Model file for the job. Use its own axes, mm. A direction names the side the tool comes from. Give positions to 0.01 mm unless a question says otherwise; leave off trailing zeros. Loops run counter-clockwise (first coordinate to the right, second up) from the corner with the lowest first, then second, coordinate; pieces in that order, holes last. Notation, with made-up numbers: (78, 2.5) - (128, 2.5) arc R12 ccw to (128, 21.5) - close; hole circle Ø4 at (52.25, -16.5). An arc over 180 degrees is marked (long way). Answer as CSV lines item,"result". Start each with the question number.
Item 1: Saw through at A-A on z = 9. Give the cut face in (x, y), plus the area to 3 significant figures.
Item 2: Drill centre lines: L1, parallel to X at y = 1.05, z = 15.99; L2, parallel to X at y = 6.5, z = -15.5; L3, parallel to Z at x = -8.65, y = 6.2. Where is each one in solid material? Low to high. Write a range as from..to.
Item 3: Saw through at D-D on y = 5.5. State how many separate pieces and enclosed holes the cut face has, plus the area to 3 significant figures.
Item 4: Saw through at B-B on x = 0. Give the cut face in (y, z).
Item 5: Tool access for faces 1 (the cylindrical face through (9.01, 9.25, 17.07)), 2 (the flat face through (9, 3, 17.5)), 3 (the flat face through (-9, 9.7, 0)), 4 (the flat face through (0, 2, 1)), 5 (the flat face through (-9, 3, 17.5)): list every direction of +Z, -Z, +X, -X, +Y, -Y with a clear straight run to the whole face (end or side of a thin tool).
Item 6: Saw through at C-C on z = 13.4. Give the cut face in (x, y), plus the area to 3 significant figures.
Item 7: Pull direction Y, two halves, no side cores. Call faces 6 (the cylindrical face through (8.986, 6.336, 0.215)), 7 (the flat face through (-10, 2.6, 0.2)), 8 (the cylindrical face through (9.01, 9.27, -17.05)): pulls with the +Y half, pulls with the -Y half, needs draft (parallel to the pull), parting line crosses it, or undercut.
Item 8: Pin check, flat tips, straight feed: pin 1 (3 mm diameter, centred on x = 0, z = 15.99, fed in from +Y); pin 2 (2 mm diameter, centred on x = 7, y = 2.5, fed in from +Z); pin 3 (6 mm diameter, centred on x = 3.5, z = -12.5, fed in from +Y). Stop position of each tip, or through.
from build123d import *

# Parameters (mm, degrees)
IZIM1_W                     = 16
IZIM1_H                     = 35
IZIM1_R                     = 1.65
Y_KSEKLIK_EKSTR_ZYON1_DEPTH = 2
IZIM3_W                     = 2
IZIM3_H                     = 35
Y_KSEKLIK_EKSTR_ZYON2_DEPTH = 9.7
RADYUS1_R                   = 1.5
KES_EKSTR_ZYON1_DEPTH       = 2
KES_EKSTR_ZYON1_2_DEPTH     = 2
KES_EKSTR_ZYON1_START       = -20
KES_EKSTR_ZYON1_3_OUTLINE_R = 1.65
KES_EKSTR_ZYON1_3_DEPTH     = 20


# Read off the part's stored shape, not the designer's step: Kes-Ekstrüzyon1
with BuildPart() as part:
    # Çizim1 → Yükseklik-Ekstrüzyon1 (new body)
    with BuildSketch(Plane(origin=(0, 0, 0), x_dir=(1, 0, 0), z_dir=(0, 1, 0))):
        Rectangle(IZIM1_W, IZIM1_H)
        with Locations(Location((0, -9, 0), (0, 0, 270))):
            Circle(IZIM1_R, mode=Mode.SUBTRACT)
        with Locations(Location((0, 9, 0), (0, 0, 270))):
            Circle(IZIM1_R, mode=Mode.SUBTRACT)
    extrude(amount=Y_KSEKLIK_EKSTR_ZYON1_DEPTH)

    # Çizim3 → Yükseklik-Ekstrüzyon2 (add)
    with BuildSketch(Plane(origin=(0, 0, 0), x_dir=(1, 0, 0), z_dir=(0, 1, 0))):
        with Locations((9, 0)):
            Rectangle(IZIM3_W, IZIM3_H)
        with Locations((-9, 0)):
            Rectangle(IZIM3_W, IZIM3_H)
    extrude(amount=Y_KSEKLIK_EKSTR_ZYON2_DEPTH)

    # Radyus1
    radyus1_edges = [part.edges().sort_by_distance(p)[0] for p in [
        (9, 9.7, 17.5),
        (9, 9.7, -17.5),
        (-9, 9.7, 17.5),
        (-9, 9.7, -17.5),
    ]]
    fillet(radyus1_edges, radius=RADYUS1_R)

    # Kes-Ekstrüzyon1 outline → Kes-Ekstrüzyon1 (add)
    with BuildSketch(Plane(origin=(0, 0, 0), x_dir=(1, 0, 0), z_dir=(0, 1, 0))):
        with BuildLine():
            ThreePointArc((0.665131566, -17.5), (0, -17.64), (-0.665131566, -17.5))
            Line((-0.665131566, -17.5), (-3, -17.5))
            ThreePointArc((-3, -17.5), (0, -19.348586012), (3, -17.5))
            Line((3, -17.5), (0.665131566, -17.5))
        make_face()
    extrude(amount=KES_EKSTR_ZYON1_DEPTH)

    # Kes-Ekstr_zyon1 2 outline → Kes-Ekstr_zyon1 2 (cut)
    with BuildSketch(Plane(origin=(0, 0, 0), x_dir=(1, 0, 0), z_dir=(0, 1, 0))):
        with BuildLine():
            ThreePointArc((0.665131566, -17.5), (0, -14.34), (-0.665131566, -17.5))
            Line((-0.665131566, -17.5), (0.665131566, -17.5))
        make_face()
    extrude(amount=KES_EKSTR_ZYON1_2_DEPTH, mode=Mode.SUBTRACT)

    # Kes-Ekstr_zyon1 3 outline → Kes-Ekstr_zyon1 3 (cut)
    with BuildSketch(Plane(origin=(10, 0, 0), x_dir=(0, 0, -1), z_dir=(1, 0, 0)).offset(KES_EKSTR_ZYON1_START)):
        with Locations((-13.4, 6.2)):
            Circle(KES_EKSTR_ZYON1_3_OUTLINE_R)
        with Locations((0, 4.7)):
            Circle(KES_EKSTR_ZYON1_3_OUTLINE_R)
        with Locations((13.4, 6.2)):
            Circle(KES_EKSTR_ZYON1_3_OUTLINE_R)
    extrude(amount=KES_EKSTR_ZYON1_3_DEPTH, mode=Mode.SUBTRACT)


solid = part.part
Responses:
1,outline,"(-10, 0) - (-1.65, 0) - (-1.65, 2) - (-8, 2) - (-8, 9.7) - (-10, 9.7) - close; (1.65, 0) - (10, 0) - (10, 9.7) - (8, 9.7) - (8, 2) - (1.65, 2) - close"
1,area,"64.2 mm2"
2,L1,"-10..-1.65, 1.65..10"
2,L2,"-10..-8, 8..10"
2,L3,"-17.5..-15.05, -11.75..-0.69, 0.69..11.75, 15.05..17.5"
3,separate pieces,"8"
3,enclosed holes,"0"
3,area,"105 mm2"
4,outline,"(0, -17.5) - (2, -17.5) - (2, -10.65) - (0, -10.65) - close; (0, -7.35) - (2, -7.35) - (2, 7.35) - (0, 7.35) - close; (0, 10.65) - (2, 10.65) - (2, 14.34) - (0, 14.34) - close; (0, 17.64) - (2, 17.64) - (2, 19.35) - (0, 19.35) - close"
5,face 1,"+Z, +X, -X, +Y"
5,face 2,"+Z, +X, +Y, -Y"
5,face 3,"+Z, -Z, +X, -X, +Y"
5,face 4,"+Z, -Z, +Y"
5,face 5,"+Z, -X, +Y, -Y"
6,outline,"(-10, 0) - (10, 0) - (10, 4.55) - (8, 4.55) - (8, 2) - (-8, 2) - (-8, 4.55) - (-10, 4.55) - close; (-10, 7.85) - (-8, 7.85) - (-8, 9.7) - (-10, 9.7) - close; (8, 7.85) - (10, 7.85) - (10, 9.7) - (8, 9.7) - close"
6,area,"57.6 mm2"
7,face 6,"undercut"
7,face 7,"needs draft"
7,face 8,"pulls with the +Y half"
8,pin 1,"through"
8,pin 2,"z = 17.5"
8,pin 3,"y = 2"
